Part print with two shaded views. Sizes in mm from the minimum x, y, z corner. Coordinates: 2 decimals unless noted, no trailing zeros. Write each loop counter-clockwise with the first axis right and the second up, starting at its lowest first coordinate (ties: lowest second). Pieces come first, ordered by that corner, then holes.
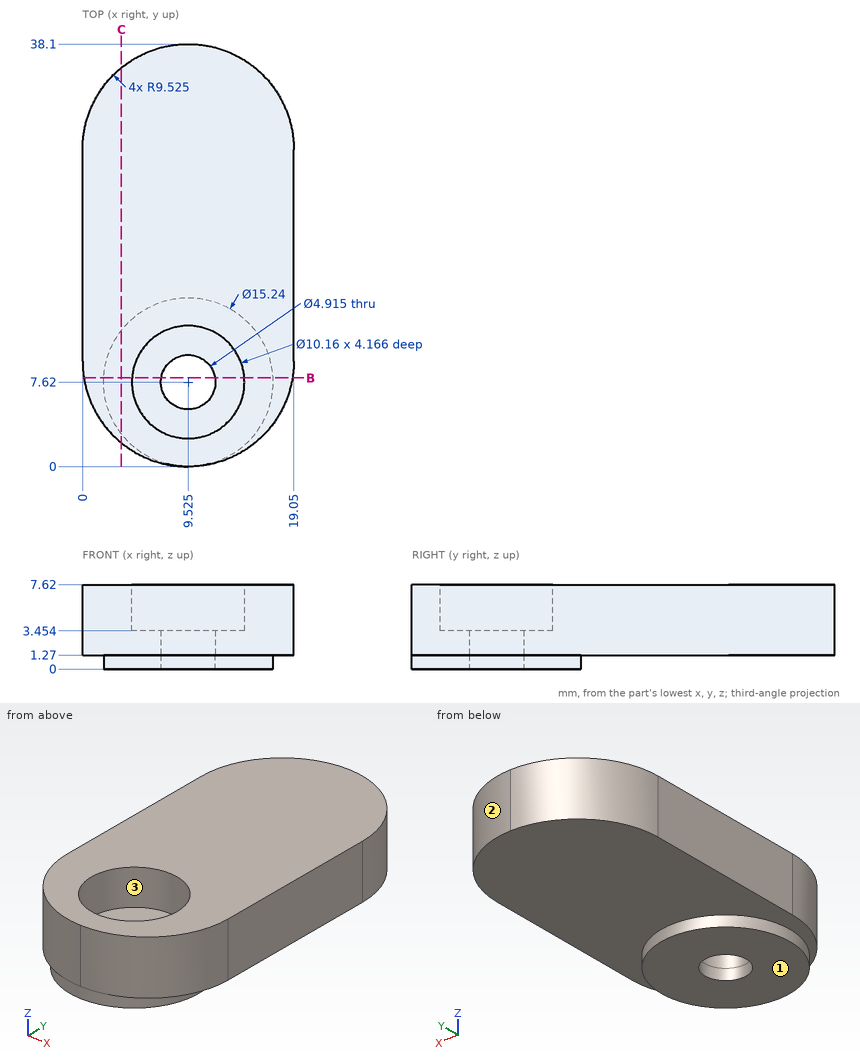
(1) Probe L1, parallel to Y at x = 6.5, z = 4.5 (1 decimal); L2, parallel to X at y = 8.5, z = 1.75 (1 decimal); L3, parallel to Z at x = 9.75, y = 3 (1 decimal). List the from-to ranges inside material, lowest first.
(2) Slice it at B-B, the plane y = 8. List the corners of the cut face in (x, z) (1 decimal).
(3) Slice it at C-C, the plane x = 3.5. List the corners of the cut face in (y, z) (1 decimal).
(4) Two-plate mould, pull along X, no slides. Class the marked faces 1, 2 and 3: pulls with the +X half, pulls with the -X half, needs draft (parallel to the pull), parting line crosses it, or undercut.
(5) Flat gauge pins, fed straight in: P1, Ø3, axis at x = 2.5, y = 16, coming from the -Z side; P2, Ø8, axis at x = 9.525, y = 7.62, coming from the -Z side; P3, Ø4.5, axis at x = 9.525, y = 7.62, coming from the +Z side; P4, Ø1, axis at x = 3.5, z = 4.5, coming from the -Y side (1 decimal). Where does each tip first touch, or does it go through?
Results:
1. L1: y = 0.5 to 3.5, 11.7 to 37.6
1. L2: x = 0.1 to 7.2, 11.8 to 19
1. L3: z = 0 to 3.5
2. outline: (0.1, 1.3) - (1.9, 1.3) - (1.9, 0) - (7.1, 0) - (7.1, 3.5) - (4.5, 3.5) - (4.5, 7.6) - (0.1, 7.6) - close; (12, 0) - (17.1, 0) - (17.1, 1.3) - (18.9, 1.3) - (18.9, 7.6) - (14.6, 7.6) - (14.6, 3.5) - (12, 3.5) - close
3. outline: (2.1, 1.3) - (3, 1.3) - (3, 0) - (12.3, 0) - (12.3, 1.3) - (36, 1.3) - (36, 7.6) - (2.1, 7.6) - close
4. face 1: needs draft
4. face 2: pulls with the +X half
4. face 3: undercut
5. P1: stops at z = 1.27
5. P2: stops at z = 0
5. P3: passes through
5. P4: stops at y = 1.8
